Check sheet for the drawn part. Datum: minimum x, y, z corner. Units: mm. Round coordinates to 2 decimals unless told otherwise and drop trailing zeros. Write each loop counter-clockwise with the first axis right and the second up, starting at its lowest first coordinate (ties: lowest second). Pieces come first, ordered by that corner, then holes. Notation, with made-up numbers: (-2.75, 75) - (30.25, 75) arc R26 ccw to (30.25, 99) - close; hole circle Ø7 at (44, 40.5). An arc over 180 degrees is marked (long way). Answer as a JSON object with one key per item and string values.
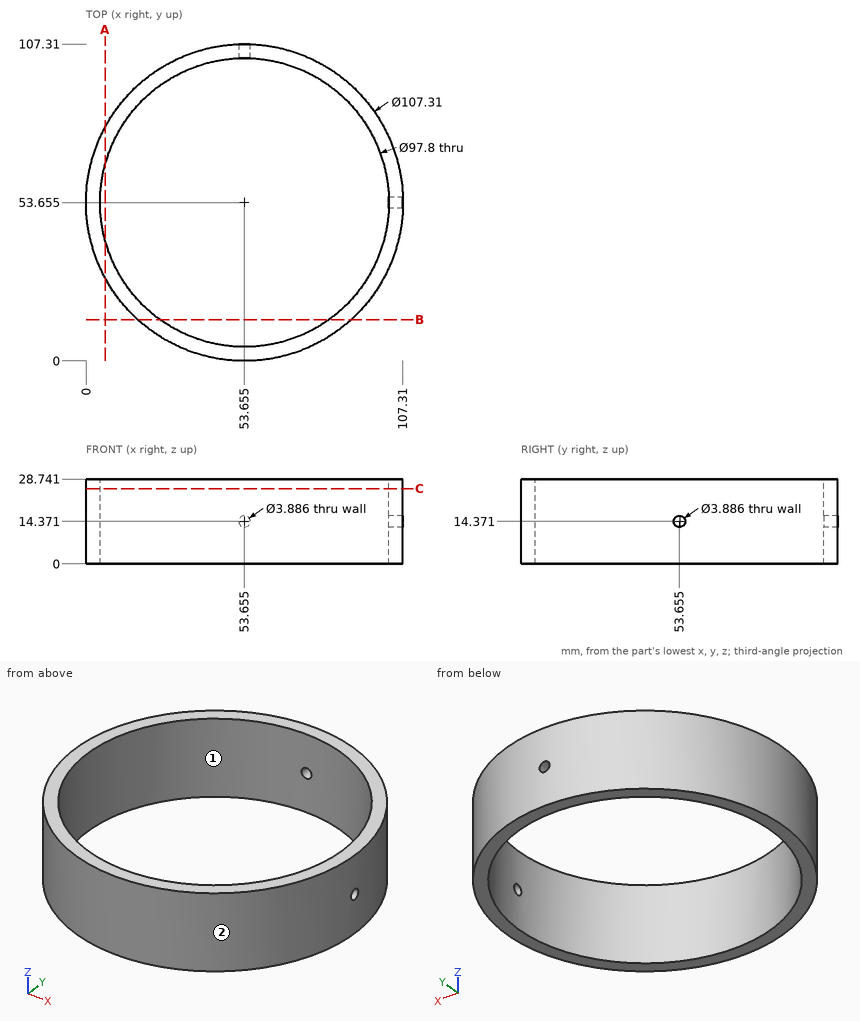
Q1. Section check A-A, the plane x = 6.5. Record the cut outline in (y, z), then the cut area to 3 significant figures.
Geometry check:
{"outline": "(28.06, 0) - (40.71, 0) - (40.71, 28.74) - (28.06, 28.74) - close; (66.6, 0) - (79.25, 0) - (79.25, 28.74) - (66.6, 28.74) - close", "area": "727 mm2"}
Q2. Section check C-C, the plane z = 25.5. Record the cut outline in (x, y) (1 decimal).
Geometry check:
{"outline": "circle Ø107.3 at (53.7, 53.7); hole circle Ø97.8 at (53.7, 53.7)"}
Q3. Section check B-B, the plane y = 14. Record the cut outline in (x, z), then the cut area to 3 significant figures.
Geometry check:
{"outline": "(17.51, 0) - (25.04, 0) - (25.04, 28.74) - (17.51, 28.74) - close; (82.27, 0) - (89.8, 0) - (89.8, 28.74) - (82.27, 28.74) - close", "area": "433 mm2"}
Q4. Gauge pin test, flat ends, axial feed: P1, Ø1.5, axis at y = 54, z = 22.5, coming from the -X side; P2, Ø5, axis at x = 33, z = 13, coming from the -Y side (1 decimal); P3, Ø5, axis at y = 76.5, z = 4, coming from the +X side. Record the tip position at first contact, or that the pin passes through.
Geometry check:
{"P1": "stops at x = 0", "P2": "stops at y = 3.2", "P3": "stops at x = 103.3"}
Q5. Material ranges on line 1 along X through (y, z) = (63.5, 12) (1 decimal); line 2 along Y through (x, z) = (41.5, 10.75) (1 decimal); line 3 along Y through (x, z) = (22.5, 1.5) (1 decimal), recorded low to high. Write a range as [from, to].
Geometry check:
{"line 1": "x = [0.9, 5.8], [101.6, 106.4]", "line 2": "y = [1.4, 6.3], [101, 105.9]", "line 3": "y = [10, 16], [91.3, 97.3]"}
Q6. Release check for a two-part mould opening along X. For the marked faces 1 and 2 record: released by +X, released by -X, zero draft, split by the parting line, or undercut.
Geometry check:
{"face 1": "undercut", "face 2": "split by the parting line"}
